Source: CAD feature listing. Evaluate the final solid. Frame: model axes, mm. A direction names the side the tool comes from. Give positions to 0.01 mm unless a question says otherwise; leave off trailing zeros. Order: outer loops, then holes, each group sorted by start corner. A loop starts at its lowest first (then second) coordinate and runs counter-clockwise, first axis right, second up. Notation, with made-up numbers: (-39, -6.75) - (-19, -6.75) arc R7 ccw to (-19, -0.75) - close; hole circle Ø4 at (23.25, -13.75). An arc over 180 degrees is marked (long way). Write each question's results on one line, items separated by ' | '. Start each with the question number.
Item 1: Section D-D on x = 35.5. Output: boundary loops of the cut face in (y, z), and give its area (3 significant figures).
Item 2: Contact query for flat-ended pins moving along their axis: pin 1 Ø5 at (x, z) = (26.5, -30.5) entering from +Y; pin 2 Ø3.5 at (x, z) = (36.84, -39.18) entering from -Y; pin 3 Ø0.5 at (x, y) = (-2, 22.5) entering from +Z. Output: stop coordinate, or through.
Item 3: Mould query, pull axis X, two halves, no side actions, for faces 1 (the flat face through (39.51, 15.776, -41.815)), 2 (the cylindrical face through (39.19, 0.99, -27.81)), 3 (the flat face through (3, 32, -37)). Classes: released by +X, released by -X, zero draft, split by the parting line, or undercut.
Item 4: Section B-B on x = 22. Output: boundary loops of the cut face in (y, z), and give its area (3 significant figures).
Item 5: Set-up query: faces 4 (the cylindrical face through (1.19, 1.01, -41.41)), 5 (the cylindrical face through (8.55, 31.51, -32.09)), 6 (the cylindrical face through (-1.91, 31.507, -32.113)), 7 (the cylindrical face through (29.752, 31.507, -42.549)), 8 (the flat face through (19, 6, -42.5)). Return all of +Z, -Z, +X, -X, +Y, -Y with unobstructed straight access to the full face (end or side cutting, diameter ignored); none if empty.
Item 6: Section A-A on y = 15. State how many separate pieces and enclosed holes the cut face has, and give its area (3 significant figures).
Item 7: Section C-C on z = -5. Output: boundary loops of the cut face in (x, y).
Item 8: Line query: line 1 along X through (y, z) = (4.5, -32); line 2 along Z through (x, y) = (18.5, 10); line 3 along X through (y, z) = (21.5, -39). Output: solid intervals per line, ascending.
```python
from build123d import *

# Parameters (mm, degrees)
SKETCH1_R           = 21
BOSS_EXTRUDE1_DEPTH = 2
BOSS_EXTRUDE6_DEPTH = 30
SKETCH13_W          = 30.324405
SKETCH13_H          = 0.5
SKETCH13_W_2        = 0.5
SKETCH13_H_2        = 30.324404
SKETCH13_W_3        = 30.32440476
SKETCH13_H_3        = 0.50000019
BOSS_EXTRUDE7_DEPTH = 9
SKETCH15_R          = 1.35
BOSS_EXTRUDE9_DEPTH = 1
SKETCH16_R          = 2.25
CUT_EXTRUDE1_DEPTH  = 3


with BuildPart() as part:
    # Sketch1 → Boss-Extrude1 (new body)
    with BuildSketch(Plane(origin=(0, 0, 0), x_dir=(1, 0, 0), z_dir=(0, 1, 0))):
        Polygon((0, 0), (38.32440476, 0), (40.66220238, 2.33779762), (40.66220238, 40.66220238), (38.32440476, 43), (0, 43), (-2.33779762, 40.66220238), (-2.33779762, 2.33779762), align=None)
        with Locations((19.16220238, 21.5)):
            Circle(SKETCH1_R, mode=Mode.SUBTRACT)
    extrude(amount=BOSS_EXTRUDE1_DEPTH)

    # Sketch3 → Boss-Extrude6 (add)
    with BuildSketch(Plane(origin=(0, 2, 0), x_dir=(1, 0, 0), z_dir=(0, 1, 0))):
        Polygon((34.324405, 1), (34.324405, 0), (38.32440476, 0), (40.66220238, 2.33779762), (40.66220238, 6.337798), (39.66220238, 6.337798), (39.66220238, 3.33779738), (37.324405, 1), align=None)
        Polygon((-2.33779762, 2.33779762), (0, 0), (4, 0), (4, 1), (1, 1), (-1.33779762, 3.337798), (-1.33779762, 6.337798), (-2.33779762, 6.337798), align=None)
        Polygon((-2.33779762, 40.66220238), (-2.33779762, 36.662202), (-1.33779762, 36.662202), (-1.33779762, 39.662202), (1, 41.99999962), (4, 41.99999962), (4, 43), (0, 43), align=None)
        Polygon((39.66220238, 39.662202), (37.32440476, 41.99999962), (34.32440476, 41.99999962), (34.32440476, 43), (38.32440476, 43), (40.66220238, 40.66220238), (40.66220238, 36.662202), (39.66220238, 36.662202), align=None)
    extrude(amount=BOSS_EXTRUDE6_DEPTH)

    # Sketch13 → Boss-Extrude7 (add)
    with BuildSketch(Plane(origin=(0, 2, 0), x_dir=(1, 0, 0), z_dir=(0, 1, 0))):
        with Locations((19.1622025, 0.25)):
            Rectangle(SKETCH13_W, SKETCH13_H)
        with Locations((-2.08779762, 21.5)):
            Rectangle(SKETCH13_W_2, SKETCH13_H_2)
        with Locations((40.41220238, 21.5)):
            Rectangle(SKETCH13_W_2, SKETCH13_H_2)
        with Locations((19.16220238, 42.749999905)):
            Rectangle(SKETCH13_W_3, SKETCH13_H_3)
    extrude(amount=BOSS_EXTRUDE7_DEPTH)

    # Sketch15 → Boss-Extrude9 (add)
    with BuildSketch(Plane(origin=(0, 32, 0), x_dir=(1, 0, 0), z_dir=(0, 1, 0))):
        with BuildLine():
            Line((4, 0), (7.5, 0))
            ThreePointArc((7.5, 0), (8.560660172, 0.439339828), (9, 1.5))
            Line((9, 1.5), (9, 9.837798))
            ThreePointArc((9, 9.837798), (8.560660172, 10.898458172), (7.5, 11.337798))
            Line((7.5, 11.337798), (-0.83779762, 11.337798))
            ThreePointArc((-0.83779762, 11.337798), (-1.898457792, 10.898458172), (-2.33779762, 9.837798))
            Line((-2.33779762, 9.837798), (-2.33779762, 6.337798))
            Line((-2.33779762, 6.337798), (-2.33779762, 2.33779762))
            Line((-2.33779762, 2.33779762), (0, 0))
            Line((0, 0), (4, 0))
        make_face()
        with Locations((6.78783338, 9.125631)):
            Circle(SKETCH15_R, mode=Mode.SUBTRACT)
        with BuildLine():
            Line((39.16220238, 11.337798), (30.82440476, 11.337798))
            ThreePointArc((30.82440476, 11.337798), (29.763744588, 10.898458172), (29.32440476, 9.837798))
            Line((29.32440476, 9.837798), (29.32440476, 1.5))
            ThreePointArc((29.32440476, 1.5), (29.763744588, 0.439339828), (30.82440476, 0))
            Line((30.82440476, 0), (34.32440476, 0))
            Line((34.32440476, 0), (38.32440476, 0))
            Line((38.32440476, 0), (40.66220238, 2.33779762))
            Line((40.66220238, 2.33779762), (40.66220238, 6.337798))
            Line((40.66220238, 6.337798), (40.66220238, 9.837798))
            ThreePointArc((40.66220238, 9.837798), (40.222862552, 10.898458172), (39.16220238, 11.337798))
        make_face()
        with Locations((31.53657138, 9.125631)):
            Circle(SKETCH15_R, mode=Mode.SUBTRACT)
        with BuildLine():
            Line((-0.83779762, 31.662202), (7.5, 31.662202))
            ThreePointArc((7.5, 31.662202), (8.560660172, 32.101541828), (9, 33.162202))
            Line((9, 33.162202), (9, 41.5))
            ThreePointArc((9, 41.5), (8.560660172, 42.560660171), (7.5, 43))
            Line((7.5, 43), (4, 43))
            Line((4, 43), (0, 43))
            Line((0, 43), (-2.33779762, 40.66220238))
            Line((-2.33779762, 40.66220238), (-2.33779762, 36.662202))
            Line((-2.33779762, 36.662202), (-2.33779762, 33.162202))
            ThreePointArc((-2.33779762, 33.162202), (-1.898457792, 32.101541828), (-0.83779762, 31.662202))
        make_face()
        with Locations((6.78783338, 33.874369)):
            Circle(SKETCH15_R, mode=Mode.SUBTRACT)
        with BuildLine():
            Line((40.66220238, 36.662202), (40.66220238, 33.162202))
            ThreePointArc((40.66220238, 33.162202), (40.222862552, 32.101541828), (39.16220238, 31.662202))
            Line((39.16220238, 31.662202), (30.82440476, 31.662202))
            ThreePointArc((30.82440476, 31.662202), (29.763744588, 32.101541828), (29.32440476, 33.162202))
            Line((29.32440476, 33.162202), (29.32440476, 41.5))
            ThreePointArc((29.32440476, 41.5), (29.763744588, 42.560660171), (30.82440476, 43))
            Line((30.82440476, 43), (34.32440476, 43))
            Line((34.32440476, 43), (38.32440476, 43))
            Line((38.32440476, 43), (40.66220238, 40.66220238))
            Line((40.66220238, 40.66220238), (40.66220238, 36.662202))
        make_face()
        with Locations((31.53657138, 33.874369)):
            Circle(SKETCH15_R, mode=Mode.SUBTRACT)
    extrude(amount=-BOSS_EXTRUDE9_DEPTH)

    # Sketch16 → Cut-Extrude1 (cut, through all)
    with BuildSketch(Plane(origin=(0, 2, 0), x_dir=(1, 0, 0), z_dir=(0, 1, 0))):
        with Locations((36.83987191, 39.177669529)):
            Circle(SKETCH16_R)
        with Locations((36.83987191, 3.82233047)):
            Circle(SKETCH16_R)
        with Locations((1.48453285, 3.82233047)):
            Circle(SKETCH16_R)
        with Locations((1.48453285, 39.177669529)):
            Circle(SKETCH16_R)
    extrude(amount=-CUT_EXTRUDE1_DEPTH, mode=Mode.SUBTRACT)


solid = part.part
```
Evaluation:
1) outline: (0, -43) - (32, -43) - (32, -31.66) - (31, -31.66) - (31, -42) - (2, -42) - (2, -40.99) - (0, -40.99) - close; (0, -37.37) - (2, -37.37) - (2, -34.69) - (0, -34.69) - close; (0, -8.31) - (2, -8.31) - (2, -5.63) - (0, -5.63) - close; (0, -2.01) - (2, -2.01) - (2, -1) - (31, -1) - (31, -11.34) - (32, -11.34) - (32, 0) - (0, 0) - close | area: 99.4 mm^2
2) pin 1: passes through | pin 2: stops at y = 31 | pin 3: stops at z = -1.75
3) face 1: released by +X | face 2: undercut | face 3: zero draft
4) outline: (0, -43) - (11, -43) - (11, -42.5) - (2, -42.5) - (2, -42.31) - (0, -42.31) - close; (0, -0.69) - (2, -0.69) - (2, -0.5) - (11, -0.5) - (11, 0) - (0, 0) - close | area: 11.8 mm^2
5) face 4: -Y | face 5: +Y, -Y | face 6: -X, +Y | face 7: -Z, +Y | face 8: none
6) separate pieces: 4 | enclosed holes: 0 | area: 46.7 mm^2
7) outline: (-2.34, 0) - (-0.43, 0) - (-0.43, 2) - (-1.34, 2) - (-1.34, 31) - (9, 31) - (9, 32) - (-2.34, 32) - close; (3.4, 0) - (6.17, 0) - (6.17, 2) - (3.4, 2) - close; (29.32, 31) - (39.66, 31) - (39.66, 2) - (38.76, 2) - (38.76, 0) - (40.66, 0) - (40.66, 32) - (29.32, 32) - close; (32.15, 0) - (34.92, 0) - (34.92, 2) - (32.15, 2) - close
8) line 1: x = -2.34 to -1.84, 40.16 to 40.66 | line 2: z = -43 to -42.5, -0.5 to 0 | line 3: x = -2.34 to -1.34, 39.66 to 40.66
